The listing builds one solid part. Answer for the finished solid, in the listing's coordinates (mm). Face numbers are marked on the shaded views. Coordinates: 2 decimals unless noted, no trailing zeros. Write each loop counter-clockwise with the first axis right and the second up, starting at its lowest first coordinate (ties: lowest second). Pieces come first, ordered by that corner, then holes. Notation, with made-up numbers: M 69.5,-13.75 L 82.5,-13.75 A25 cw 82.5,24.25 Z; hole C 72.25,51 d3. An arc over 180 degrees is marked long. Answer as CSV lines item,"result". Start each with the question number.
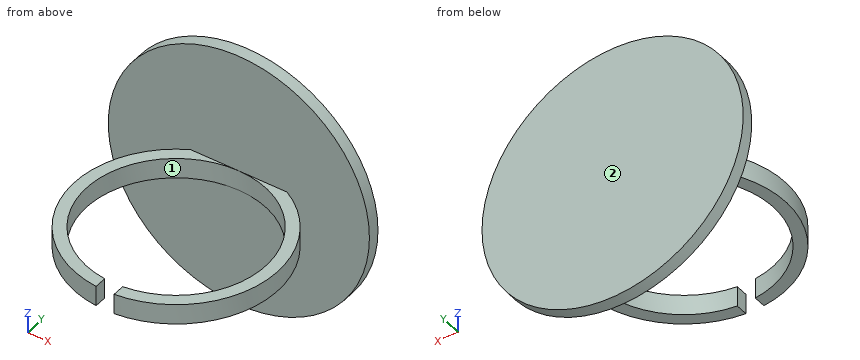
```python
from build123d import *

# Parameters (mm, degrees)
ESQUISSE1_R             = 32.139129067
BOSS_EXTRU_1_DEPTH      = 3
ESQUISSE2_R             = 25
BOSS_EXTRU_2_DEPTH      = 2.5
BOSS_EXTRU_2_DEPTH_BACK = 2.5
ESQUISSE3_R             = 22
ENL_V_MAT_EXTRU_1_DEPTH = 5
ESQUISSE7_W             = 4.438304304
ESQUISSE7_H             = 8.275677871
ENL_V_MAT_EXTRU_4_DEPTH = 5


with BuildPart() as part:
    # Esquisse1 → Boss.-Extru.1 (new body)
    with BuildSketch(Plane(origin=(0, 0, 0), x_dir=(1, 0, 0), z_dir=(0, 1, 0))):
        Circle(ESQUISSE1_R)
    extrude(amount=BOSS_EXTRU_1_DEPTH)

    # Esquisse2 → Boss.-Extru.2 (add, two sides)
    with BuildSketch(Plane.XY) as boss_extru_2_sk:
        with Locations((0, -22)):
            Circle(ESQUISSE2_R)
    extrude(amount=BOSS_EXTRU_2_DEPTH)
    extrude(boss_extru_2_sk.sketch, amount=-BOSS_EXTRU_2_DEPTH_BACK)

    # Esquisse3 → Enl_v. mat.-Extru.1 (cut)
    with BuildSketch(Plane.XY.offset(2.5)):
        with Locations((0, -22)):
            Circle(ESQUISSE3_R)
    extrude(amount=-ENL_V_MAT_EXTRU_1_DEPTH, mode=Mode.SUBTRACT)

    # Esquisse7 → Enl_v. mat.-Extru.4 (cut)
    with BuildSketch(Plane.XY.offset(2.5)):
        with Locations((0, -45.862161065)):
            Rectangle(ESQUISSE7_W, ESQUISSE7_H)
    extrude(amount=-ENL_V_MAT_EXTRU_4_DEPTH, mode=Mode.SUBTRACT)


solid = part.part
```
1) The part is cut by section B-B (x = -13.5). Determine the outline of the cut face in (y, z), then the cut area to 3 significant figures.
2) The part is cut by section A-A (y = -4). Determine the outline of the cut face in (x, z), then the cut area to 3 significant figures.
3) For a pull along X with two mould halves and no side action, classify the marked faces 1 and 2 as +X half, -X half, draft (parallel to the pull), parting line (faces both ways), or undercut.
4) The part is cut by section C-C (y = -25.5). Determine the outline of the cut face in (x, z).
5) Each of these flat-tipped pins is pushed along its axis until it touches: P1, Ø6, axis at x = -3, z = 15, coming from the -Y side; P2, Ø10, axis at y = -20, z = 12, coming from the -X side; P3, Ø7.5, axis at x = 16.5, y = -31, coming from the -Z side; P4, Ø20, axis at x = -10.5, y = -28.5, coming from the +Z side. Where does it stop, or does it pass through?
6) The part is cut by section D-D (z = 0). Determine the outline of the cut face in (x, y).
7) Find the intervals of material crossed by line 1 (X direction, y = -22, z = 1); line 2 (Y direction, x = 20, z = -22.5); line 3 (X direction, y = -29.5, z = 1), in increasing order. Write a range as from..to.
Completed:
1,outline,"M -43.04,-2.5 L -39.37,-2.5 L -39.37,2.5 L -43.04,2.5 Z; M -4.63,-2.5 L -0.96,-2.5 L -0.96,2.5 L -4.63,2.5 Z; M 0,-29.17 L 3,-29.17 L 3,29.17 L 0,29.17 Z"
1,area,"212 mm²"
2,outline,"M -17.35,-2.5 L -12.65,-2.5 L -12.65,2.5 L -17.35,2.5 Z; M 12.65,-2.5 L 17.35,-2.5 L 17.35,2.5 L 12.65,2.5 Z"
2,area,"47.0 mm²"
3,face 1,"undercut"
3,face 2,"draft"
4,outline,"M -24.75,-2.5 L -21.72,-2.5 L -21.72,2.5 L -24.75,2.5 Z; M 21.72,-2.5 L 24.75,-2.5 L 24.75,2.5 L 21.72,2.5 Z"
5,P1,"y = 0"
5,P2,"through"
5,P3,"z = -2.5"
5,P4,"z = 2.5"
6,outline,"M -32.14,0 L -11.87,0 A25 ccw -2.22,-46.9 L -2.22,-43.89 A22 cw long 2.22,-43.89 L 2.22,-46.9 A25 ccw 11.87,0 L 32.14,0 L 32.14,3 L -32.14,3 Z"
7,line 1,"-25..-22, 22..25"
7,line 2,"0..3"
7,line 3,"-23.85..-20.68, 20.68..23.85"
